from build123d import *

# Parameters (mm, degrees)
SKETCH_W     = 20
SKETCH_H     = 20
SKETCH_W_2   = 14
SKETCH_H_2   = 14
PAD_DEPTH    = 50
SKETCH002_W  = 20
SKETCH002_H  = 20
PAD001_DEPTH = 30
POCKET_DEPTH = 20.001


with BuildPart() as part:
    # Sketch → Pad (new body)
    with BuildSketch(Plane.XY):
        Rectangle(SKETCH_W, SKETCH_H)
        Rectangle(SKETCH_W_2, SKETCH_H_2, mode=Mode.SUBTRACT)
    extrude(amount=PAD_DEPTH)

    # Sketch002 (on Face9 of Pad) → Pad001 (join)
    with BuildSketch(Plane(origin=(0, 0, 0), x_dir=(1, 0, 0), z_dir=(0, 0, -1))):
        Rectangle(SKETCH002_W, SKETCH002_H)
    extrude(amount=PAD001_DEPTH)

    # Sketch003 (on Face7 of Pad001) → Pocket (cut, through all)
    with BuildSketch(Plane(origin=(-10, 0, 0), x_dir=(0, -1, 0), z_dir=(-1, 0, 0))):
        Polygon((-10, -10), (10, -21.547005), (10, -30), (-10, -30), align=None)
    extrude(amount=-POCKET_DEPTH, mode=Mode.SUBTRACT)


solid = part.part
Read the model definition and answer for the solid it produces. Units are mm, in the model's axes. A direction names the side the tool comes from. Coordinates: 2 decimals unless noted, no trailing zeros. Loops run counter-clockwise (first coordinate to the right, second up) from the corner with the lowest first, then second, coordinate; pieces in that order, holes last. Notation, with made-up numbers: (66.25, -26) -> (93.25, -26) arc R29 cw to (93.25, 13) -> close; hole circle Ø9 at (0.5, -30). An arc over 180 degrees is marked (long way). Write item = value, one per line. Start each with the question number.
1) The mould has two halves that part along X. Classify faces 1 (the face through (0, -10, 15)), 2 (the face through (0, -7, 25)), 3 (the face through (-10, 0, 15)): pulls with the +X half, pulls with the -X half, needs draft (parallel to the pull), parting line crosses it, or undercut.
2) The part is cut by section C-C, the plane y = 4.5. Determine the outline of the cut face in (x, z).
3) The part is cut by section A-A, the plane z = 25.5. Determine the outline of the cut face in (x, y).
4) Find the intervals of material crossed by L1, parallel to X at y = -6.5, z = 5.5; L2, parallel to Z at x = -2.25, y = -8, in increasing order. Write a range as from..to.
5) The part is cut by section D-D, the plane z = -16. Determine the outline of the cut face in (x, y), plus the area to 3 significant figures.
6) Given P1, Ø5, axis at x = -0.5, y = -0.5, coming from the -Z side; P2, Ø11, axis at x = 0, y = 0.5, coming from the +Z side, each flat-ended and moving along its own axis, determine where each tip first touches the part or whether it passes through.
7) The part is cut by section B-B, the plane x = -1.25. Determine the outline of the cut face in (y, z), plus the area to 3 significant figures.
8) For faces 4 (the face through (0, 0, 0)), 5 (the face through (0, 10, 20)), determine the directions among +Z, -Z, +X, -X, +Y, -Y from which every point of the face is accessible in a straight line to the end or side of a thin tool.
Result:
q1.face_1 = needs draft
q1.face_2 = undercut
q1.face_3 = pulls with the -X half
q2.outline = (-10, -13.18) -> (10, -13.18) -> (10, 50) -> (7, 50) -> (7, 0) -> (-7, 0) -> (-7, 50) -> (-10, 50) -> close
q3.outline = (-10, -10) -> (10, -10) -> (10, 10) -> (-10, 10) -> close; hole (-7, -7) -> (7, -7) -> (7, 7) -> (-7, 7) -> close
q4.L1 = -10..-7, 7..10
q4.L2 = -20.39..50
q5.outline = (-10, -10) -> (10, -10) -> (10, -0.39) -> (-10, -0.39) -> close
q5.area = 192 mm²
q6.P1 = -17.51
q6.P2 = 0
q7.outline = (-10, -21.55) -> (10, -10) -> (10, 50) -> (7, 50) -> (7, 0) -> (-7, 0) -> (-7, 50) -> (-10, 50) -> close
q7.area = 615 mm²
q8.face_4 = +Z
q8.face_5 = +Z, -Z, +X, -X, +Y
